Autodesk Inventor part; units mm, degrees
ref_plane "Arbeitsebene1" through (0, 28.95, 0) normal (0, 1, 0) x (-1, 0, 0)
ref_plane "YZ Plane" through (0, 0, 0) normal (1, 0, 0) x (0, 1, 0)
ref_plane "XY Plane" through (0, 0, 0) normal (0, 0, 1) x (1, 0, 0)
sketch "Skizze1" plane through (0, 0, 0) normal (0, 0, 1) x (1, 0, 0)
  line L0 (-90, -65.25) -> (90, -65.25)
  line L1 (90, -65.25) -> (90, 65.25)
  line L2 (90, 65.25) -> (-90, 65.25)
  line L3 (-90, 65.25) -> (-90, -65.25)
  line L4 (-90, -65.25) -> (90, 65.25) construction
  line L5 (90, -65.25) -> (-90, 65.25) construction
  point P0 (0, 0)
  dimension "d0" = 180
  dimension "d1" = 130.5
extrude "Extrusion1" add sketch "Skizze1" along normal blind 0.8
sketch "Skizze2" plane through (0, 0, 0.8) normal (0, 0, 1) x (1, 0, 0)
  line L0 (90, -65.25) -> (90, 65.25)
  line L1 (90, 65.25) -> (-90, 65.25)
  line L2 (-90, 65.25) -> (-90, -65.25)
  line L3 (-90, -65.25) -> (90, -65.25)
  line L4 (-85, 60.25) -> (85, 60.25)
  line L5 (85, 60.25) -> (85, -60.25)
  line L6 (85, -60.25) -> (-85, -60.25)
  line L7 (-85, -60.25) -> (-85, 60.25)
  point P0 (0, 0)
  dimension "d4" = 5
extrude "Extrusion2" add sketch "Skizze2" along normal blind 3.2
ref_plane "Arbeitsebene1" through (0, 28.95, 0) normal (0, 1, 0) x (-1, 0, 0)
sketch "Skizze4" plane through (0, 28.95, 0) normal (0, 1, 0) x (-1, 0, 0)
  line L0 (0, 0) -> (0, 5.6907) construction
  line L1 (-85, 0.8) -> (85, 0.8)
  line L2 (31.5, 0.8) -> (35, 0.8)
  line L3 (35, 8.4503) -> (31.5, 8.4503)
  line L4 (35, 8.4503) -> (35, 0.8)
  line L5 (31.5, 8.4503) -> (31.5, 6.8503)
  line L6 (31.5, 6.8503) -> (33, 5.8)
  line L7 (33, 5.8) -> (31.5, 6.8503)
  line L8 (33, 5.8) -> (33, 4.2)
  line L9 (33, 4.2) -> (31.5, 4.2)
  line L10 (31.5, 4.2) -> (31.5, 0.8)
  line L11 (-90, 0) -> (90, 0)
  dimension "d8" = 33
  dimension "d9" = 1.6
  dimension "d11" = 125
  dimension "d12" = 1.5
  dimension "d13" = 1.6
  dimension "d14" = 2
  dimension "d17" = 4.2
extrude "Extrusion3" add sketch "Skizze4" along normal up to surface (31.3 mm away)
sketch "Skizze5" plane through (-35, 60.25, 4) normal (0, 1, 0) x (1, 0, 0)
  line L0 (0, -4.4503) -> (3.5, -4.4503)
  line L1 (2, -0.2) -> (3.5, -0.2)
  line L2 (3.5, -4.4503) -> (3.5, -0.2)
  line L3 (3.5, -0.2) -> (0, -0.2)
  line L4 (0, 3.2) -> (0, -4.4503)
  line L5 (0, -0.2) -> (0, -4.4503)
  line L6 (0, -4.4503) -> (3.5, -4.4503)
  point P0 (35, 4)
  point P1 (0, -0.2)
  point P2 (0, 4.4503)
  point P3 (3.5, 4.4503)
  point P4 (2, 0.2)
  point P5 (3.5, 0.2)
  point P6 (0, 0)
  point P7 (0, -3.2)
extrude "Extrusion4" add sketch "Skizze5" against normal blind 0.8
mirror "Spiegeln1" about plane through (0, 0, 0) normal (1, 0, 0) of "Extrusion3", "Extrusion4"
sketch "Skizze6" plane through (0, 0, 0.8) normal (0, 0, 1) x (1, 0, 0)
  line L0 (-31.5, 28.95) -> (-35, 28.95)
  line L1 (31.5, 28.95) -> (31.5, 60.25)
  line L2 (-31.5, 28.95) -> (31.5, 28.95)
  line L3 (31.5, 28.95) -> (31.5, 36.95)
  line L4 (31.5, 36.95) -> (-31.5, 36.95)
  line L5 (-31.5, 36.95) -> (-31.5, 28.95)
  point P0 (0, 0)
  dimension "d20" = 8
extrude "Extrusion5" cut sketch "Skizze6" against normal up to surface (0.8 mm away)
sketch "Skizze7" plane through (85, 60.25, 0.8) normal (0, -1, 0) x (1, 0, 0)
  line L0 (0, 0) -> (-50, 0)
  line L1 (-47.2, 0) -> (-47.2, 0.2)
  line L2 (-47.2, 0.2) -> (-49.6, 0.2)
  line L3 (-49.6, 0.2) -> (-49.6, 5.2)
  line L4 (5, 3.2) -> (-175, 3.2)
  line L5 (-49.6, 5.2) -> (-47.2, 6.8805)
  line L6 (-47.2, 6.8805) -> (-47.2, 7.6503)
  line L7 (-47.2, 7.6503) -> (-51.5, 7.6503)
  line L8 (-51.5, 7.6503) -> (-51.5, 0)
  line L9 (-51.5, 0) -> (-47.2, 0)
  line L10 (-50, 0) -> (-50, 7.6503)
  line L11 (-50, 7.6503) -> (-53.5, 7.6503)
  point P0 (-85, -0.8)
  point P1 (-50, 3.2)
  dimension "d23" = 0.2
  dimension "d24" = 5
  dimension "d25" = 125
  dimension "d26" = 2.4
  dimension "d31" = 1.5
  dimension "d32" = 0.4
extrude "Extrusion6" add sketch "Skizze7" along normal blind 61.2
ref_plane "Arbeitsebene2" through (54.2, 60.25, 6) normal (1, 0, 0) x (0, 0, -1)
mirror "Spiegeln2" about plane through (54.2, 60.25, 6) normal (1, 0, 0) of "Extrusion6"
sketch "Skizze8" plane through (0, 0, 0.8) normal (0, 0, 1) x (1, 0, 0)
  circle A0 centre (-86.5, -3.75) radius 3
  circle A1 centre (-33.4, -3.75) radius 3
  circle A2 centre (-33.4, -27.55) radius 3
  circle A3 centre (-86.5, -27.55) radius 3
  line L0 (-33.4, -27.55) -> (-33.4, -3.75) construction
  line L1 (-35, 28.95) -> (-35, 60.25)
  line L2 (-35, 28.95) -> (-35, -60.25) construction
  line L3 (85, -60.25) -> (-85, -60.25)
  line L4 (-33.4, -15.65) -> (-35, -15.65) construction
  line L5 (-90, 65.25) -> (-90, -65.25)
  point P0 (0, 0)
  dimension "d33" = 53.1
  dimension "d34" = 23.8
  dimension "d35" = 6
  dimension "d36" = 3.5
extrude "Extrusion7" add sketch "Skizze8" along normal blind 3.2
sketch "Skizze9" plane through (-33.4, -3.75, 4) normal (0, 0, 1) x (1, 0, 0)
  circle A0 centre (0, 0) radius 3
  circle A1 centre (0, -23.8) radius 3
  arc A2 (-51.6, -2.5981) -> (-51.6, 2.5981) centre (-53.1, 0) ccw
  arc A3 (-51.6, -26.3981) -> (-51.6, -21.2019) centre (-53.1, -23.8) ccw
  point P0 (33.4, 3.75)
hole "Bohrung1" at (-33.4, -3.75, 4) at (-33.4, -27.55, 4) at (-86.5, -3.75, 4) at (-86.5, -27.55, 4) direction (0, 0, -1) diameter 3.2 end through all
fillet "Rundung1" radius 2 4 edges at (-83.5, -3.75, 0.8) (-83.5, -27.55, 0.8) (-36.4, -27.55, 0.8) (-36.4, -3.75, 0.8)
fillet "Rundung2" radius 7 4 edges at (-85, 60.25, 2.4) (85, 60.25, 2.4) (85, -60.25, 2.4) (-85, -60.25, 2.4)
sketch "Skizze10" plane through (0, 0, 4) normal (0, 0, 1) x (1, 0, 0)
  line L0 (90, 65.25) -> (-90, 65.25)
  line L1 (-90, 65.25) -> (-90, -65.25)
  point P0 (0, 0)
  point P1 (-85.5, 60.75)
  dimension "d48" = 4.5
  dimension "d49" = 4.5
hole "Bohrung2" at (-85.5, 60.75, 4) direction (0, 0, -1) diameter 3.2 depth 15
mirror "Spiegeln3" about plane through (0, 0, 0) normal (1, 0, 0) of "Bohrung2"
mirror "Spiegeln4" about plane through (0, 0, 0) normal (0, 1, 0) of "Bohrung2", "Spiegeln3"
properties part number "Back Cover v5"
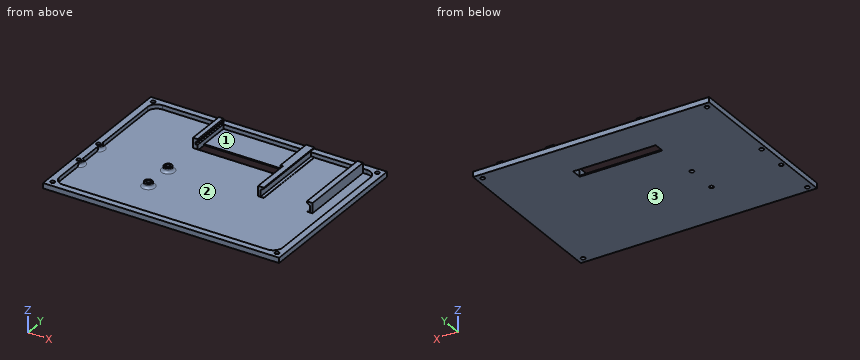
Input: part model. Units: mm. Frame: model coordinates. Face numbers are marked on the shaded views. Round coordinates to 2 decimals unless told otherwise and drop trailing zeros. Loops run counter-clockwise (first coordinate to the right, second up) from the corner with the lowest first, then second, coordinate; pieces in that order, holes last. Notation, with made-up numbers: (25.5, 13) - (48.5, 13) arc R16 cw to (48.5, 33) - close; hole circle Ø10 at (17.5, 72). An arc over 180 degrees is marked (long way). One line per item, written item: value. Start each with the question number.
(1) Ray query, line 1 (X direction, y = 15, z = 3.25); line 2 (X direction, y = 60.75, z = 2.95); line 3 (Y direction, x = -33.4, z = 2.85). Return the intervals inside material, ascending. Write a range as [from, to].
(2) Draft query along Y for the marked faces 1, 2 and 3. Return one class per face: +Y half, -Y half, draft (parallel to the pull), parting line (faces both ways), or undercut.
(3) Section C-C, the plane y = 22. Return loops of the section in (x, z).
(4) Contact query for flat-ended pins moving along their axis: P1, Ø0.8, axis at x = -32.5, z = 5.5, coming from the -Y side; P2, Ø4, axis at x = -34, z = 6.5, coming from the +Y side; P3, Ø4, axis at x = -33.4, y = -3.75, coming from the +Z side. Output: stop coordinate, or through.
(5) Section B-B, the plane x = -73. Return loops of the section in (y, z), plus the area to 3 significant figures.
(6) Section A-A, the plane y = -37.5. Return loops of the section in (x, z).
Results below:
1. line 1: [-90, -85], [33.5, 35.4], [73, 74.9], [85, 90]
1. line 2: [-90, -87.1], [-83.9, 83.9], [87.1, 90]
1. line 3: [-65.25, -60.25], [-30.55, -29.15], [-25.95, -24.55], [-6.75, -5.35], [-2.15, -0.75], [28.95, 65.25]
2. face 1: undercut
2. face 2: undercut
2. face 3: draft
3. outline: (-90, 0) - (90, 0) - (90, 4) - (85, 4) - (85, 0.8) - (74.9, 0.8) - (74.9, 8.45) - (70.6, 8.45) - (70.6, 7.68) - (73, 6) - (73, 1) - (70.6, 1) - (70.6, 0.8) - (37.8, 0.8) - (37.8, 1) - (35.4, 1) - (35.4, 6) - (37.8, 7.68) - (37.8, 8.45) - (33.5, 8.45) - (33.5, 0.8) - (-85, 0.8) - (-85, 4) - (-90, 4) - close
4. P1: y = 59.45
4. P2: y = 60.25
4. P3: z = 4
5. outline: (-65.25, 0) - (65.25, 0) - (65.25, 4) - (60.25, 4) - (60.25, 0.8) - (-60.25, 0.8) - (-60.25, 4) - (-65.25, 4) - close
5. area: 136 mm^2
6. outline: (-90, 0) - (90, 0) - (90, 4) - (85, 4) - (85, 0.8) - (-85, 0.8) - (-85, 4) - (-90, 4) - close
